Here's how the part is built. I have some questions about the finished solid (model axes, mm). Coordinates: 2 decimals unless noted, no trailing zeros. Order: outer loops, then holes, each group sorted by start corner. A loop starts at its lowest first (then second) coordinate and runs counter-clockwise, first axis right, second up. Notation, with made-up numbers: (89.5, 13) - (106.5, 13) arc R11 cw to (106.5, 18) - close; hole circle Ø7 at (-8.5, 54). An arc over 180 degrees is marked (long way). Answer in a Markdown table with one row per item. Add a question column.
Item 1: I want a section at B-B (z = 81). Count the separate pieces of the cut face and the enclosed holes in it, plus the area to 3 significant figures.
Item 2: Will this pin go through, and if not, where does the flat tip stop? pin 1 Ø24 at (x, z) = (1812, 81) entering from +Y.
Item 3: Thinking about a two-plate mould opening in X: for faces 1 (the cylindrical face through (1830.475, -2.465, 73.34)), 2 (the flat face through (1168, -5, 100)), which applies, +X half, -X half, draft (parallel to the pull), parting line (faces both ways), or undercut?
Item 4: If I drill on line 1 along Z through (x, y) = (2126, -1.25); line 2 along Z through (x, y) = (1341, -2.1), over which ranges is the centre line in solid material (lowest first)? Write a range as from..to.
Item 5: I want a section at A-A (x = 1969). Please give me the cut outline in (y, z).
```python
from build123d import *

# Parameters (mm, degrees)
F0_R     = 20
F1_DEPTH = 5


with BuildPart() as f1:
    # F0 (on Front) → F1 (new body)
    with BuildSketch(Plane.XZ):
        with BuildLine():
            ThreePointArc((2106, 0), (2126, 20), (2146, 0))
            Line((2146, 0), (2370, 0))
            Line((2370, 0), (2370, 162))
            Line((2370, 162), (2146, 162))
            ThreePointArc((2146, 162), (2126, 142), (2106, 162))
            Line((2106, 162), (1832, 162))
            ThreePointArc((1832, 162), (1812, 142), (1792, 162))
            Line((1792, 162), (1518, 162))
            ThreePointArc((1518, 162), (1498, 142), (1478, 162))
            Line((1478, 162), (1205, 162))
            ThreePointArc((1205, 162), (1185, 142), (1165, 162))
            Line((1165, 162), (890, 162))
            ThreePointArc((890, 162), (870, 142), (850, 162))
            Line((850, 162), (576, 162))
            ThreePointArc((576, 162), (556, 142), (536, 162))
            Line((536, 162), (262, 162))
            ThreePointArc((262, 162), (242, 142), (222, 162))
            Line((222, 162), (0, 162))
            Line((0, 162), (0, 0))
            Line((0, 0), (222, 0))
            ThreePointArc((222, 0), (242, 20), (262, 0))
            Line((262, 0), (536, 0))
            ThreePointArc((536, 0), (556, 20), (576, 0))
            Line((576, 0), (850, 0))
            ThreePointArc((850, 0), (870, 20), (890, 0))
            Line((890, 0), (1165, 0))
            ThreePointArc((1165, 0), (1185, 20), (1205, 0))
            Line((1205, 0), (1478, 0))
            ThreePointArc((1478, 0), (1498, 20), (1518, 0))
            Line((1518, 0), (1792, 0))
            ThreePointArc((1792, 0), (1812, 20), (1832, 0))
            Line((1832, 0), (2106, 0))
        make_face()
        with Locations((85, 81)):
            Circle(F0_R, mode=Mode.SUBTRACT)
        with Locations((242, 81)):
            Circle(F0_R, mode=Mode.SUBTRACT)
        with Locations((399, 81)):
            Circle(F0_R, mode=Mode.SUBTRACT)
        with Locations((556, 81)):
            Circle(F0_R, mode=Mode.SUBTRACT)
        with Locations((713, 81)):
            Circle(F0_R, mode=Mode.SUBTRACT)
        with Locations((870, 81)):
            Circle(F0_R, mode=Mode.SUBTRACT)
        with Locations((1027, 81)):
            Circle(F0_R, mode=Mode.SUBTRACT)
        with Locations((1184, 81)):
            Circle(F0_R, mode=Mode.SUBTRACT)
        with Locations((1341, 81)):
            Circle(F0_R, mode=Mode.SUBTRACT)
        with Locations((1498, 81)):
            Circle(F0_R, mode=Mode.SUBTRACT)
        with Locations((1655, 81)):
            Circle(F0_R, mode=Mode.SUBTRACT)
        with Locations((1812, 81)):
            Circle(F0_R, mode=Mode.SUBTRACT)
        with Locations((1969, 81)):
            Circle(F0_R, mode=Mode.SUBTRACT)
        with Locations((2126, 81)):
            Circle(F0_R, mode=Mode.SUBTRACT)
        with Locations((2283, 81)):
            Circle(F0_R, mode=Mode.SUBTRACT)
    extrude(amount=F1_DEPTH)


solid = f1.part
```
Values follow:
| question | item | result |
|---|---|---|
| 1 | separate pieces | 16 |
| 1 | enclosed holes | 0 |
| 1 | area | 8,850 mm^2 |
| 2 | pin 1 | passes through |
| 3 | face 1 | undercut |
| 3 | face 2 | draft |
| 4 | line 1 | z = 20..61, 101..142 |
| 4 | line 2 | z = 0..61, 101..162 |
| 5 | outline | (-5, 0) - (0, 0) - (0, 61) - (-5, 61) - close; (-5, 101) - (0, 101) - (0, 162) - (-5, 162) - close |
